Build history of the part. All positions in model axes, mm. Face numbers are marked on the shaded views. A direction names the side the tool comes from. Coordinates: 2 decimals unless noted, no trailing zeros. Order: outer loops, then holes, each group sorted by start corner. A loop starts at its lowest first (then second) coordinate and runs counter-clockwise, first axis right, second up. Notation, with made-up numbers: (41.25, -5.75) - (62.25, -5.75) arc R14 cw to (62.25, 2.25) - close; hole circle Ø10 at (23, 12.25). An arc over 180 degrees is marked (long way). Answer as CSV lines item,"result". Start each with the question number.
from build123d import *

# Parameters (mm, degrees)
F0_W     = 31.75
F0_H     = 31.75
F0_R     = 2.0955
F0_R_2   = 12.7
F1_DEPTH = 7.62
F0_R_3   = 6.35
F2_DEPTH = 38.1
F3_R     = 1.7272
F4_DEPTH = 15.875
F5_R     = 1.27


with BuildPart() as f1:
    # F0 (on Top) → F1 (new body)
    with BuildSketch(Plane.XY):
        with Locations((15.875, 15.875)):
            Rectangle(F0_W, F0_H)
        with Locations((4.064, 4.064)):
            Circle(F0_R, mode=Mode.SUBTRACT)
        with Locations((27.686, 4.064)):
            Circle(F0_R, mode=Mode.SUBTRACT)
        with Locations((4.064, 27.686)):
            Circle(F0_R, mode=Mode.SUBTRACT)
        with Locations((15.875, 15.875)):
            Circle(F0_R_2, mode=Mode.SUBTRACT)
        with Locations((27.686, 27.686)):
            Circle(F0_R, mode=Mode.SUBTRACT)
    extrude(amount=F1_DEPTH)

    # F0 (on Top) → F2 (join)
    with BuildSketch(Plane.XY):
        with Locations((15.875, 15.875)):
            Circle(F0_R_2)
        with Locations((15.875, 15.875)):
            Circle(F0_R_3, mode=Mode.SUBTRACT)
    extrude(amount=F2_DEPTH)

    # F3 (on Front) → F4 (cut)
    with BuildSketch(Plane.XZ):
        with Locations((15.875, 13.97)):
            Circle(F3_R)
        with Locations((15.875, 33.02)):
            Circle(F3_R)
    extrude(amount=-F4_DEPTH, mode=Mode.SUBTRACT)

    # F5
    f5_edges = [f1.edges().sort_by_distance(p)[0] for p in [
        (3.175, 15.875, 38.1),
        (9.525, 15.875, 38.1),
    ]]
    fillet(f5_edges, radius=F5_R)


solid = f1.part
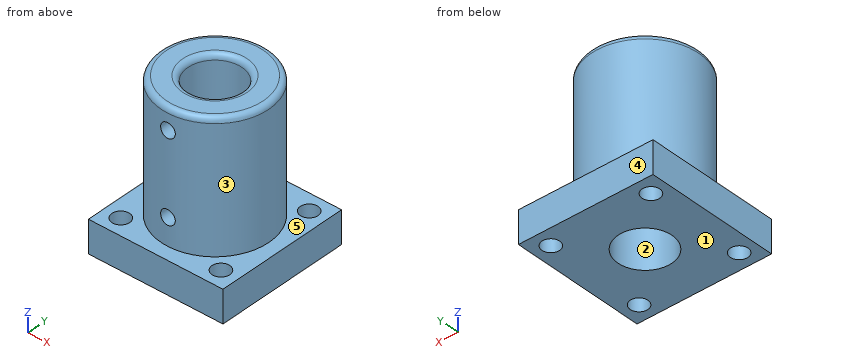
(1) Probe L1, parallel to Y at x = 29, z = 5; L2, parallel to Z at x = 30.5, y = 18.5; L3, parallel to Z at x = 17, y = 6. List the from-to ranges inside material, lowest first. Write a range as [from, to].
(2) Which spindle directions (+Z, -Z, +X, -X, +Y, -Y) get a long thin tool onto all of the face, cutting with end or side? Do the marked faces 4 and 5. Say none if no direction does.
(3) Drop flat-ended pins along their axis: pin 1 Ø1.5 at (x, y) = (12.5, 5) entering from -Z; pin 2 Ø5 at (x, z) = (7.5, 12.5) entering from +Y; pin 3 Ø4 at (x, z) = (15.875, 33.02) entering from -Y (3 decimals); pin 4 Ø1 at (y, z) = (23, 12.5) entering from -X. Give the stop position or say it passes through.
(4) Band-saw the part on B-B on z = 13.97. List the corners of the cut face in (x, y) (3 decimals), plus the area to 3 significant figures.
(5) Pull direction X, two halves, no side cores. Call the marked faces 1, 2 and 3: +X half, -X half, draft (parallel to the pull), parting line (faces both ways), or undercut.
(6) Band-saw the part on A-A on z = 9. List the corners of the cut face in (x, y) (3 decimals).
Filled in:
1,L1,"y = [0, 2.43], [5.7, 26.05], [29.32, 31.75]"
1,L2,"z = [0, 7.62]"
1,L3,"z = [0, 12.66], [15.28, 31.71], [34.33, 38.1]"
2,face 4,"+Z, -Z, +X, -X, +Y"
2,face 5,"+Z"
3,pin 1,"stops at z = 0"
3,pin 2,"stops at y = 27.13"
3,pin 3,"stops at y = 3.175"
3,pin 4,"stops at x = 5.04"
4,outline,"(14.148, 3.293) - (14.148, 9.764) arc R6.35 cw (long way) to (17.602, 9.764) - (17.602, 3.293) arc R12.7 ccw (long way) to start"
4,area,"358 mm^2"
5,face 1,"draft"
5,face 2,"undercut"
5,face 3,"parting line"
6,outline,"circle Ø25.4 at (15.875, 15.875); hole circle Ø12.7 at (15.875, 15.875)"
